Build history of the part. All positions in model axes, mm. A direction names the side the tool comes from. Round coordinates to 2 decimals unless told otherwise and drop trailing zeros. Loops run counter-clockwise (first coordinate to the right, second up) from the corner with the lowest first, then second, coordinate; pieces in that order, holes last. Notation, with made-up numbers: M 22.25,-27.5 L 78.25,-27.5 A28 ccw 78.25,-1.5 Z; hole C -2.75,30.25 d6. An arc over 180 degrees is marked long. One line per item, written item: value.
```python
from build123d import *

# Parameters (mm, degrees)
BOSS_EXTRUDE1_DEPTH                        = 15
BOSS_EXTRUDE2_START                        = 6
SKETCH1_3_R                                = 6
BOSS_EXTRUDE2_DEPTH                        = 9
BOSS_EXTRUDE3_START                        = -15
SKETCH1_4_R                                = 6
BOSS_EXTRUDE3_DEPTH                        = 9
FILLET1_RADIUS                             = 15
FILLET1_LENGTH                             = 9
FILLET2_RADIUS                             = 15
FILLET2_LENGTH                             = 9
F_12_0MM_DOWEL_HOLE1_D                     = 12
F_12_0MM_DOWEL_HOLE1_CSINK_D               = 12.05
F_12_0MM_DOWEL_HOLE1_CSINK_ANGLE           = 90
F_12_0MM_DOWEL_HOLE1_ON_FACE_2_D           = 12
F_12_0MM_DOWEL_HOLE1_ON_FACE_2_CSINK_D     = 12.05
F_12_0MM_DOWEL_HOLE1_ON_FACE_2_CSINK_ANGLE = 90
FILLET3_R                                  = 3
FILLET4_R                                  = 3
FILLET5_R                                  = 1


with BuildPart() as part:
    # Sketch1 → Boss-Extrude1 (new, symmetric)
    with BuildSketch(Plane.XY):
        Polygon((0, 45), (0, 0), (9, 0), (9, 36), (60, 36), (60, 45), (30, 45), align=None)
    extrude(amount=BOSS_EXTRUDE1_DEPTH, both=True)

    # Sketch1<3> → Boss-Extrude2 (add)
    with BuildSketch(Plane.XY.offset(BOSS_EXTRUDE2_START)):
        with BuildLine():
            Line((0, 60), (0, 45))
            Line((0, 45), (30, 45))
            Line((30, 45), (30, 60))
            ThreePointArc((30, 60), (15, 75), (0, 60))
        make_face()
        with Locations((15, 60)):
            Circle(SKETCH1_3_R, mode=Mode.SUBTRACT)
    extrude(amount=BOSS_EXTRUDE2_DEPTH)

    # Sketch1<4> → Boss-Extrude3 (add)
    with BuildSketch(Plane.XY.offset(BOSS_EXTRUDE3_START)):
        with BuildLine():
            Line((0, 60), (0, 45))
            Line((0, 45), (30, 45))
            Line((30, 45), (30, 60))
            ThreePointArc((30, 60), (15, 75), (0, 60))
        make_face()
        with Locations((15, 60)):
            Circle(SKETCH1_4_R, mode=Mode.SUBTRACT)
    extrude(amount=BOSS_EXTRUDE3_DEPTH)

    # Fillet1: full round fillet: the end face becomes a half cylinder, R = half its width
    fillet1_face = Plane((60, 40.5, 0), x_dir=(0, -1, 0), z_dir=(1, 0, 0))  # on the end face: x along it, z out of the body
    fillet1_slab = fillet1_face.offset(-FILLET1_RADIUS / 2) * Box(FILLET1_LENGTH, 2 * FILLET1_RADIUS, FILLET1_RADIUS, mode=Mode.PRIVATE)  # the body's end, R deep
    fillet1_round = Plane((45, 40.5, 0), x_dir=(1, 0, 0), z_dir=(0, -1, 0)) * Cylinder(FILLET1_RADIUS, FILLET1_LENGTH, mode=Mode.PRIVATE)  # its axis R under the face
    add(fillet1_slab - fillet1_round, mode=Mode.SUBTRACT)

    # Fillet2: full round fillet: the end face becomes a half cylinder, R = half its width
    fillet2_face = Plane((4.5, 0, 0), x_dir=(-1, 0, 0), z_dir=(0, -1, 0))  # on the end face: x along it, z out of the body
    fillet2_slab = fillet2_face.offset(-FILLET2_RADIUS / 2) * Box(FILLET2_LENGTH, 2 * FILLET2_RADIUS, FILLET2_RADIUS, mode=Mode.PRIVATE)  # the body's end, R deep
    fillet2_round = Plane((4.5, 15, 0), x_dir=(0, -1, 0), z_dir=(-1, 0, 0)) * Cylinder(FILLET2_RADIUS, FILLET2_LENGTH, mode=Mode.PRIVATE)  # its axis R under the face
    add(fillet2_slab - fillet2_round, mode=Mode.SUBTRACT)

    # Ø12.0mm Dowel Hole1 (through all)
    with Locations(Plane(origin=(9, 14.262563745, 0.728544171), x_dir=(0, 0, 1), z_dir=(1, 0, 0))):
        with Locations((0, 0)):
            CounterSinkHole(F_12_0MM_DOWEL_HOLE1_D / 2, F_12_0MM_DOWEL_HOLE1_CSINK_D / 2, counter_sink_angle=F_12_0MM_DOWEL_HOLE1_CSINK_ANGLE)

    # Ø12.0mm Dowel Hole1 on face 2 (through all)
    with Locations(Plane(origin=(45, 45, 0), x_dir=(0, 0, 1), z_dir=(0, 1, 0))):
        with Locations((0, 0)):
            CounterSinkHole(F_12_0MM_DOWEL_HOLE1_ON_FACE_2_D / 2, F_12_0MM_DOWEL_HOLE1_ON_FACE_2_CSINK_D / 2, counter_sink_angle=F_12_0MM_DOWEL_HOLE1_ON_FACE_2_CSINK_ANGLE)

    # Fillet3
    fillet3_edges = [part.edges().sort_by_distance(p)[0] for p in [
        (9, 36, 0),
    ]]
    fillet(fillet3_edges, radius=FILLET3_R)

    # Fillet4
    fillet4_edges = [part.edges().sort_by_distance(p)[0] for p in [
        (30, 45, 10.5),
        (30, 45, -10.5),
    ]]
    fillet(fillet4_edges, radius=FILLET4_R)

    # Fillet5
    fillet5_edges = [part.edges().sort_by_distance(p)[0] for p in [
        (16.5, 45, 6),
        (16.5, 45, -6),
    ]]
    fillet(fillet5_edges, radius=FILLET5_R)


solid = part.part
```
Item 1: Wall check: line 1 along Y through (x, z) = (15, -8); line 2 along Z through (x, y) = (8, 68.5); line 3 along Y through (x, z) = (47.5, 5.5). Give the ranges that are in metal, low to high.
Check values:
line 1: y = 36 to 54, 66 to 75
line 2: z = -15 to -6, 6 to 15
line 3: y = 36 to 45
Item 2: Pull direction Z, two halves, no side cores. Call faces 1 (the face through (20.54, 57.7, 10.44)), 2 (the face through (17, 45, 15)), 3 (the face through (39.143, 40.425, 1.301)): pulls with the +Z half, pulls with the -Z half, needs draft (parallel to the pull), parting line crosses it, or undercut.
Check values:
face 1: needs draft
face 2: pulls with the +Z half
face 3: undercut
Item 3: Which spindle directions (+Z, -Z, +X, -X, +Y, -Y) get a long thin tool onto all of the face, cutting with end or side? Do faces 4 (the face through (30, 54, 10)), 5 (the face through (19, 54, -6)), 6 (the face through (37, 45, 0)). Say none if no direction does.
Check values:
face 4: +Z, -Z, +X, +Y
face 5: +X, -X, +Y
face 6: +X, +Y
Item 4: Drop flat-ended pins along their axis: P1, Ø10, axis at x = 7, z = 0, coming from the +Y side; P2, Ø9, axis at x = 24, z = -1, coming from the -Y side; P3, Ø1, axis at x = 19, z = -11, coming from the +Y side; P4, Ø8.5, axis at x = 10, y = 62.5, coming from the -Z side. Give the stop position or say it passes through.
Check values:
P1: stops at y = 45
P2: stops at y = 36
P3: stops at y = 74.59
P4: stops at z = -15
Item 5: Slice it at B-B, the plane x = 24. Give the cut face in (y, z), and give its area (3 significant figures).
Check values:
outline: M 36,-15 L 72,-15 L 72,-6 L 46,-6 A1 cw 45,-5 L 45,5 A1 cw 46,6 L 72,6 L 72,15 L 36,15 Z
area: 756 mm2
Item 6: Slice it at A-A, the plane x = 15. Give the cut face in (y, z).
Check values:
outline: M 36,-15 L 54,-15 L 54,-6 L 46,-6 A1 cw 45,-5 L 45,5 A1 cw 46,6 L 54,6 L 54,15 L 36,15 Z; M 66,-15 L 75,-15 L 75,-6 L 66,-6 Z; M 66,6 L 75,6 L 75,15 L 66,15 Z
Item 7: Slice it at D-D, the plane y = 28.5. Give the cut face in (x, z).
Check values:
outline: M 0,-15 L 9,-15 L 9,15 L 0,15 Z
Item 8: Slice it at C-C, the plane z = 1. Give the number of separate pieces and of enclosed holes in the cut face, and give its area (3 significant figures).
Check values:
separate pieces: 3
enclosed holes: 0
area: 651 mm2
